from build123d import *

# Parameters (mm, degrees)
F0_W     = 6.3956826925
F0_H     = 2.5
F0_W_2   = 4.1414871812
F0_W_3   = 5.4119601846
F0_W_4   = 5.0508699417
F0_W_5   = 26
F0_H_2   = 34.8582080007
F0_R     = 3
F0_W_6   = 21
F0_H_3   = 14.1105238348
F1_DEPTH = 3
F2_DEPTH = 5
F3_DEPTH = 1.4
F5_DEPTH = 5
F7_DEPTH = 5
F8_R     = 3
F9_DEPTH = 2


with BuildPart() as f1:
    # F0 (on Top) → F1 (new body)
    with BuildSketch(Plane.XY):
        with Locations((-7.3393285275, -1.25)):
            Rectangle(F0_W, F0_H)
        with Locations((-2.0707435906, -1.25)):
            Rectangle(F0_W_2, F0_H)
        with Locations((-13.243149966, -1.25)):
            Rectangle(F0_W_3, F0_H)
        Polygon((0, 10.8894761652), (0, 0), (0, -2.5), (2.5, -2.5), (2.5, 27.5), (-23.5, 27.5), (-23.5, -2.5), (-21, -2.5), (-21, 0), (-21, 10.8894761652), (-21, 25), (0, 25), align=None)
        with Locations((-18.4745650291, -1.25)):
            Rectangle(F0_W_4, F0_H)
        with Locations((-10.5, 44.9291040003)):
            Rectangle(F0_W_5, F0_H_2)
        with Locations((-10, 54.3582080007)):
            Circle(F0_R, mode=Mode.SUBTRACT)
        with Locations((-10.5, 17.9447380826)):
            Rectangle(F0_W_6, F0_H_3)
        Polygon((-4.1414871812, 0), (0, 0), (0, 10.8894761652), (-21, 10.8894761652), (-21, 0), (-15.9491300583, 0), (-10.5371698737, 0), align=None)
    extrude(amount=-F1_DEPTH)

    # F0 (on Top) → F2 (join)
    with BuildSketch(Plane.XY):
        Polygon((0, 10.8894761652), (0, 0), (0, -2.5), (2.5, -2.5), (2.5, 27.5), (-23.5, 27.5), (-23.5, -2.5), (-21, -2.5), (-21, 0), (-21, 10.8894761652), (-21, 25), (0, 25), align=None)
        with Locations((-7.3393285275, -1.25)):
            Rectangle(F0_W, F0_H)
    extrude(amount=F2_DEPTH)

    # F0 (on Top) → F3 (join)
    with BuildSketch(Plane.XY):
        with Locations((-10.5, 17.9447380826)):
            Rectangle(F0_W_6, F0_H_3)
    extrude(amount=F3_DEPTH)

    # F4 (on face) → F5 (join)
    with BuildSketch(Plane.YZ.offset(2.5)):
        with BuildLine():
            ThreePointArc((41.5, 7), (38.5, 10), (35.5, 7))
            Line((35.5, 7), (36.75, 7))
            ThreePointArc((36.75, 7), (38.5, 8.75), (40.25, 7))
            Line((40.25, 7), (41.5, 7))
        make_face()
        with BuildLine():
            Line((35.5, 7), (35.5, 0))
            Line((35.5, 0), (41.5, 0))
            Line((41.5, 0), (41.5, 7))
            Line((41.5, 7), (40.25, 7))
            ThreePointArc((40.25, 7), (38.5, 5.25), (36.75, 7))
            Line((36.75, 7), (35.5, 7))
        make_face()
    extrude(amount=-F5_DEPTH)

    # F6 (on face) → F7 (join)
    with BuildSketch(Plane(origin=(-23.5, 0, 0), x_dir=(0, -1, 0), z_dir=(-1, 0, 0))):
        with BuildLine():
            Line((-41.5, 7), (-41.5, 0))
            Line((-41.5, 0), (-35.5, 0))
            Line((-35.5, 0), (-35.5, 7))
            Line((-35.5, 7), (-36.75, 7))
            ThreePointArc((-36.75, 7), (-38.5, 5.25), (-40.25, 7))
            Line((-40.25, 7), (-41.5, 7))
        make_face()
        with BuildLine():
            ThreePointArc((-35.5, 7), (-38.5, 10), (-41.5, 7))
            Line((-41.5, 7), (-40.25, 7))
            ThreePointArc((-40.25, 7), (-38.5, 8.75), (-36.75, 7))
            Line((-36.75, 7), (-35.5, 7))
        make_face()
    extrude(amount=-F7_DEPTH)

    # F8 (on face) → F9 (join)
    with BuildSketch(Plane(origin=(0, 0, -3), x_dir=(1, 0, 0), z_dir=(0, 0, -1))):
        with Locations((-10, -54.3582080007)):
            Circle(F8_R)
    extrude(amount=-F9_DEPTH)


solid = f1.part
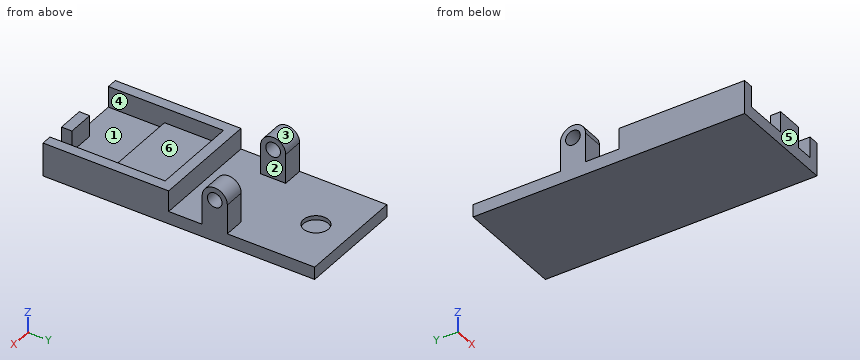
Work out the finished part from the listing and answer in its coordinate system (mm). Face numbers are marked on the shaded views. A direction names the side the tool comes from. Coordinates: 2 decimals unless noted, no trailing zeros. Write each loop counter-clockwise with the first axis right and the second up, starting at its lowest first coordinate (ties: lowest second). Pieces come first, ordered by that corner, then holes.
1. Flat-ended cylindrical pins translate along their axes: pin 1 (4 mm diameter, centred on x = -13.5, z = 6.5, fed in from -Y); pin 2 (6 mm diameter, centred on x = -6, y = 39.5, fed in from +Z); pin 3 (2.5 mm diameter, centred on x = -22, z = 4, fed in from +Y). Find the tip coordinate at first contact, or state that the pin passes through.
Results list:
pin 1: stops at y = 25
pin 2: stops at z = 0
pin 3: stops at y = 41.5
2. The part is cut by section C-C, the plane x = -19.25. Write down the section's boundary in (y, z), and give its area (3 significant figures).
Results list:
outline: (-2.5, -3) - (62.36, -3) - (62.36, 0) - (41.5, 0) - (41.5, 7) arc R3 ccw to (35.5, 7) - (35.5, 0) - (27.5, 0) - (27.5, 5) - (25, 5) - (25, 1.4) - (10.89, 1.4) - (10.89, 0) - (-2.5, 0) - close; hole circle Ø3.5 at (38.5, 7)
area: 273 mm2
3. Consider line 1 along X through (y, z) = (7, 4); line 2 along Z through (x, y) = (-20.9, 38.5); line 3 along Z through (x, y) = (-5, 52.5). Determine where each line is inside the solid, lowest interval first.
Results list:
line 1: x = -23.5 to -21, 0 to 2.5
line 2: z = -3 to 5.25, 8.75 to 10
line 3: z = -3 to 0
4. The part is cut by section A-A, the plane z = 3. Write down the section's boundary in (x, y), and give its area (3 significant figures).
Results list:
outline: (-23.5, -2.5) - (-21, -2.5) - (-21, 25) - (0, 25) - (0, -2.5) - (2.5, -2.5) - (2.5, 27.5) - (-23.5, 27.5) - close; (-23.5, 35.5) - (-18.5, 35.5) - (-18.5, 41.5) - (-23.5, 41.5) - close; (-10.54, -2.5) - (-4.14, -2.5) - (-4.14, 0) - (-10.54, 0) - close; (-2.5, 35.5) - (2.5, 35.5) - (2.5, 41.5) - (-2.5, 41.5) - close
area: 278 mm2
5. The part is cut by section D-D, the plane y = 15. Write down the section's boundary in (x, z).
Results list:
outline: (-23.5, -3) - (2.5, -3) - (2.5, 5) - (0, 5) - (0, 1.4) - (-21, 1.4) - (-21, 5) - (-23.5, 5) - close
6. For a pull along Y with two mould halves and no side action, classify the marked faces 1, 2 and 3 as +Y half, -Y half, draft (parallel to the pull), parting line (faces both ways), or undercut.
Results list:
face 1: undercut
face 2: draft
face 3: parting line
7. The part is cut by section B-B, the plane y = 38.5. Write down the section's boundary in (x, z).
Results list:
outline: (-23.5, -3) - (2.5, -3) - (2.5, 5.25) - (-2.5, 5.25) - (-2.5, 0) - (-18.5, 0) - (-18.5, 5.25) - (-23.5, 5.25) - close; (-23.5, 8.75) - (-18.5, 8.75) - (-18.5, 10) - (-23.5, 10) - close; (-2.5, 8.75) - (2.5, 8.75) - (2.5, 10) - (-2.5, 10) - close
8. For the marked faces 4, 5 and 6, determine the directions among +Z, -Z, +X, -X, +Y, -Y from which every point of the face is accessible in a straight line to the end or side of a thin tool.
Results list:
face 4: +Z, -Y
face 5: +Z, -Z, +X, -X, -Y
face 6: +Z
